Part model, mm, in its own coordinate system. Face numbers are marked on the shaded views. A direction names the side the tool comes from. Coordinates: 2 decimals unless noted, no trailing zeros. Loops run counter-clockwise (first coordinate to the right, second up) from the corner with the lowest first, then second, coordinate; pieces in that order, holes last. Notation, with made-up numbers: (11.5, 53.25) - (50.5, 53.25) arc R29 ccw to (50.5, 80.25) - close; hole circle Ø4 at (40, 47.5). An arc over 180 degrees is marked (long way). Answer as CSV lines item,"result".
from build123d import *

# Parameters (mm, degrees)
F1_DEPTH     = 8
F3_W         = 6.7527772065
F3_H         = 8
F4_DEPTH     = 4
F8_DEPTH     = 7
F9_T4_DEPTH  = 8
F9_T9_DEPTH  = 20.6550440955
F9_T15_DEPTH = 20.6550440955
F9_T21_DEPTH = 8
F9_T26_DEPTH = 20.6550440955
F9_T32_DEPTH = 20.6550440955
F12_DEPTH    = 8
F13_SIZE     = 3.5
F16_R        = 1
F17_DEPTH    = 5
F20_R        = 1
F21_DEPTH    = 5


# Not quite as in the source:
# - a fillet or chamfer that OpenCascade refuses, or shapes differently, is made with other operations: its cross-section is extruded or revolved along the edge and cut away or added


with BuildPart() as f1:
    # F0 (on Top) → F1 (new body)
    with BuildSketch(Plane.XY):
        with BuildLine():
            Line((-3.3763886032, -5.2), (3.3763886032, -5.2))
            ThreePointArc((3.3763886032, -5.2), (0, 6.2), (-3.3763886032, -5.2))
        make_face()
        with BuildLine():
            ThreePointArc((-1.8439088915, -1.2), (0, 2.2), (1.8439088915, -1.2))
            Line((1.8439088915, -1.2), (-1.8439088915, -1.2))
        make_face(mode=Mode.SUBTRACT)
    extrude(amount=F1_DEPTH)

    # F3 (on offset) → F4 (join)
    with BuildSketch(Plane.XZ.offset(5.2)):
        with Locations((0, 4)):
            Rectangle(F3_W, F3_H)
    extrude(amount=F4_DEPTH)

    # F6 (on Right) → F7 (revolve)
    with BuildSketch(Plane.YZ):
        with BuildLine():
            Line((18, 36), (18, 38))
            Line((18, 38), (1.7, 38))
            Line((1.7, 38), (1.7, 34))
            Line((1.7, 34), (0, 31.9740188926))
            Line((0, 31.9740188926), (0, 8))
            Line((0, 8), (18, 8))
            Line((18, 8), (18, 10))
            Line((18, 10), (13.7071067812, 14.2928932188))
            ThreePointArc((13.7071067812, 14.2928932188), (13.4142135624, 15), (13.7071067812, 15.7071067812))
            Line((13.7071067812, 15.7071067812), (18, 20))
            Line((18, 20), (18, 26))
            Line((18, 26), (13.7071067812, 30.2928932188))
            ThreePointArc((13.7071067812, 30.2928932188), (13.4142135624, 31), (13.7071067812, 31.7071067812))
            Line((13.7071067812, 31.7071067812), (18, 36))
        make_face()
    revolve(axis=Axis((0, 0, 19.9870094463), (0, 0, 1)))

    # F5 (on Top) → F8 (cut)
    with BuildSketch(Plane.XY):
        Polygon((3, -5.5), (3, -3), (0, -3), (-3, -3), (-3, -5.5), align=None)
    extrude(amount=F8_DEPTH, mode=Mode.SUBTRACT)

    # F9: chamfer of 7 on 2 edges, made by hand


with BuildPart() as f9_tool2:
    # F9_s3 → F9_t4 (new body)
    with BuildSketch(Plane.XY):
        with BuildLine():
            Line((-3.3002459804, -10.261444939), (-5.3591596162, -2.9755066267))
            Line((-5.3591596162, -2.9755066267), (-5.2398656841, -2.9022334545))
            ThreePointArc((-5.2398656841, -2.9022334545), (-4.424549602, -4.1408888924), (-3.3001475703, -5.0825806452))
            Line((-3.3001475703, -5.0825806452), (-3.2363886032, -5.2))
            ThreePointArc((-3.2363886032, -5.2), (-3.2363886032, -7.7307224695), (-3.1602459804, -10.261444939))
            Line((-3.1602459804, -10.261444939), (-3.3002459804, -10.261444939))
        make_face()
    extrude(amount=F9_T4_DEPTH)

    split(bisect_by=Plane.XZ.offset(9.2), keep=Keep.BOTTOM)


with BuildPart() as f1_1:
    add(f1.part)

    # F9_t1: union F9_tool2
    add(f9_tool2.part)


with BuildPart() as f9_tool7:
    # F9_s8 → F9_t9 (new body)
    with BuildSketch(Plane.XY):
        with BuildLine():
            Line((-3.3002459804, -10.261444939), (-5.3591596162, -2.9755066267))
            Line((-5.3591596162, -2.9755066267), (-5.2398656841, -2.9022334545))
            ThreePointArc((-5.2398656841, -2.9022334545), (-4.424549602, -4.1408888924), (-3.3001475703, -5.0825806452))
            Line((-3.3001475703, -5.0825806452), (-3.2363886032, -5.2))
            ThreePointArc((-3.2363886032, -5.2), (-3.2363886032, -7.7307224695), (-3.1602459804, -10.261444939))
            Line((-3.1602459804, -10.261444939), (-3.3002459804, -10.261444939))
        make_face()
    extrude(amount=F9_T9_DEPTH)

    split(bisect_by=Plane.XY.offset(8), keep=Keep.TOP)

    split(bisect_by=Plane.XZ.offset(9.2), keep=Keep.TOP)


with BuildPart() as f1_2:
    add(f1_1.part)

    # F9_t6: union F9_tool7
    add(f9_tool7.part)


with BuildPart() as f9_tool13:
    # F9_s14 → F9_t15 (new body)
    with BuildSketch(Plane.XY):
        with BuildLine():
            Line((-3.3002459804, -10.261444939), (-5.3591596162, -2.9755066267))
            Line((-5.3591596162, -2.9755066267), (-5.2398656841, -2.9022334545))
            ThreePointArc((-5.2398656841, -2.9022334545), (-4.424549602, -4.1408888924), (-3.3001475703, -5.0825806452))
            Line((-3.3001475703, -5.0825806452), (-3.2363886032, -5.2))
            ThreePointArc((-3.2363886032, -5.2), (-3.2363886032, -7.7307224695), (-3.1602459804, -10.261444939))
            Line((-3.1602459804, -10.261444939), (-3.3002459804, -10.261444939))
        make_face()
    extrude(amount=F9_T15_DEPTH)

    split(bisect_by=Plane.XY.offset(8), keep=Keep.TOP)

    split(bisect_by=Plane.XZ.offset(9.2), keep=Keep.BOTTOM)


with BuildPart() as f1_3:
    add(f1_2.part)

    # F9_t12: union F9_tool13
    add(f9_tool13.part)


with BuildPart() as f9_tool19:
    # F9_s20 → F9_t21 (new body)
    with BuildSketch(Plane.XY):
        with BuildLine():
            Line((3.3002459804, -10.261444939), (5.3591596162, -2.9755066267))
            Line((5.3591596162, -2.9755066267), (5.2398656841, -2.9022334545))
            ThreePointArc((5.2398656841, -2.9022334545), (4.424549602, -4.1408888924), (3.3001475703, -5.0825806452))
            Line((3.3001475703, -5.0825806452), (3.2363886032, -5.2))
            ThreePointArc((3.2363886032, -5.2), (3.2363886032, -7.7307224695), (3.1602459804, -10.261444939))
            Line((3.1602459804, -10.261444939), (3.3002459804, -10.261444939))
        make_face()
    extrude(amount=F9_T21_DEPTH)

    split(bisect_by=Plane.XZ.offset(9.2), keep=Keep.BOTTOM)


with BuildPart() as f1_4:
    add(f1_3.part)

    # F9_t18: union F9_tool19
    add(f9_tool19.part)


with BuildPart() as f9_tool24:
    # F9_s25 → F9_t26 (new body)
    with BuildSketch(Plane.XY):
        with BuildLine():
            Line((3.3002459804, -10.261444939), (5.3591596162, -2.9755066267))
            Line((5.3591596162, -2.9755066267), (5.2398656841, -2.9022334545))
            ThreePointArc((5.2398656841, -2.9022334545), (4.424549602, -4.1408888924), (3.3001475703, -5.0825806452))
            Line((3.3001475703, -5.0825806452), (3.2363886032, -5.2))
            ThreePointArc((3.2363886032, -5.2), (3.2363886032, -7.7307224695), (3.1602459804, -10.261444939))
            Line((3.1602459804, -10.261444939), (3.3002459804, -10.261444939))
        make_face()
    extrude(amount=F9_T26_DEPTH)

    split(bisect_by=Plane.XY.offset(8), keep=Keep.TOP)

    split(bisect_by=Plane.XZ.offset(9.2), keep=Keep.TOP)


with BuildPart() as f1_5:
    add(f1_4.part)

    # F9_t23: union F9_tool24
    add(f9_tool24.part)


with BuildPart() as f9_tool30:
    # F9_s31 → F9_t32 (new body)
    with BuildSketch(Plane.XY):
        with BuildLine():
            Line((3.3002459804, -10.261444939), (5.3591596162, -2.9755066267))
            Line((5.3591596162, -2.9755066267), (5.2398656841, -2.9022334545))
            ThreePointArc((5.2398656841, -2.9022334545), (4.424549602, -4.1408888924), (3.3001475703, -5.0825806452))
            Line((3.3001475703, -5.0825806452), (3.2363886032, -5.2))
            ThreePointArc((3.2363886032, -5.2), (3.2363886032, -7.7307224695), (3.1602459804, -10.261444939))
            Line((3.1602459804, -10.261444939), (3.3002459804, -10.261444939))
        make_face()
    extrude(amount=F9_T32_DEPTH)

    split(bisect_by=Plane.XY.offset(8), keep=Keep.TOP)

    split(bisect_by=Plane.XZ.offset(9.2), keep=Keep.BOTTOM)


with BuildPart() as f1_6:
    add(f1_5.part)

    # F9_t29: union F9_tool30
    add(f9_tool30.part)

    # F11 (on offset) → F12 (cut, through all)
    with BuildSketch(Plane.XZ.offset(9.2)):
        with BuildLine():
            ThreePointArc((0, 2.5), (1.0606601718, 2.9393398282), (1.5, 4))
            ThreePointArc((1.5, 4), (-1.0606601718, 5.0606601718), (0, 2.5))
        make_face()
    extrude(amount=-F12_DEPTH, mode=Mode.SUBTRACT)

    # F13
    f13_edges = [f1_6.edges().sort_by_distance(p)[0] for p in [
        (0, 6.2, 8),
    ]]
    chamfer(f13_edges, length=F13_SIZE)

    # F16 (on face) → F17 (cut)
    with BuildSketch(Plane(origin=(0, -1, 1), x_dir=(1, 0, 0), z_dir=(0, -0.7071067812, 0.7071067812))):
        with Locations((0, 23.2666600496)):
            Circle(F16_R)
    extrude(amount=F17_DEPTH, mode=Mode.SUBTRACT)

    # F20 (on face) → F21 (cut)
    with BuildSketch(Plane(origin=(0, -9, 9), x_dir=(1, 0, 0), z_dir=(0, -0.7071067812, 0.7071067812))):
        with Locations((0, 33.659003675)):
            Circle(F20_R)
    extrude(amount=F21_DEPTH, mode=Mode.SUBTRACT)


solid = f1_6.part
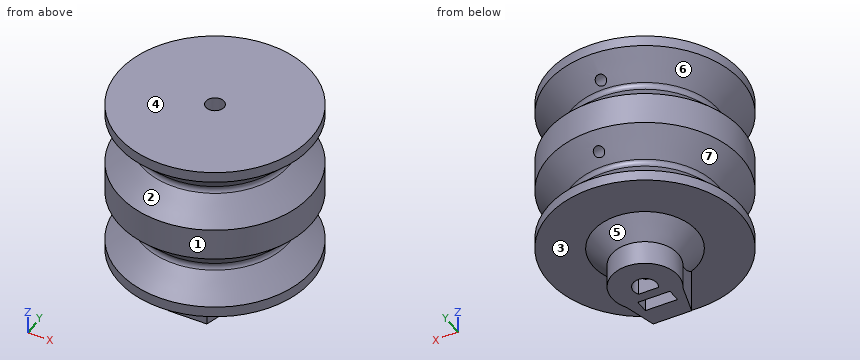
Q1. Saw through at A-A (z = 25). Give the cut face in (x, y).
Results:
outline,"circle Ø36 at (0, 0)"
Q2. Two-plate mould, pull along Z, no slides. Class the marked faces 4, 5, 6 and 7: released by +Z, released by -Z, zero draft, split by the parting line, or undercut.
Results:
face 4,"released by +Z"
face 5,"released by -Z"
face 6,"undercut"
face 7,"undercut"
Q3. Which spindle directions (+Z, -Z, +X, -X, +Y, -Y) get a long thin tool onto all of the face, cutting with end or side? Do the marked faces 1, 2 and 3. Say none if no direction does.
Results:
face 1,"+Z, -Z"
face 2,"none"
face 3,"-Z"
Q4. Wall check: L1, parallel to Z at x = 0, y = -7; L2, parallel to Y at x = 0, z = 35; L3, parallel to Y at x = -0.5, z = 2. Give the ranges that are in metal, low to high.
Results:
L1,"z = 0 to 2.5, 5.5 to 38"
L2,"y = -17 to -1.7, 1.7 to 11.19, 14.02 to 17"
L3,"y = -9.2 to -5.5, -3 to -1.2, 2.14 to 6.18"
Q5. Flat gauge pins, fed straight in: pin 1 (2 mm diameter, centred on y = -4, z = 3, fed in from -X); pin 2 (3 mm diameter, centred on x = -3.5, z = 25, fed in from +Y); pin 3 (2 mm diameter, centred on x = -0.5, z = 3, fed in from -Y). Where does each tip first touch, or does it go through?
Results:
pin 1,"stops at x = -5.43"
pin 2,"stops at y = 17.89"
pin 3,"stops at y = -9.2"
